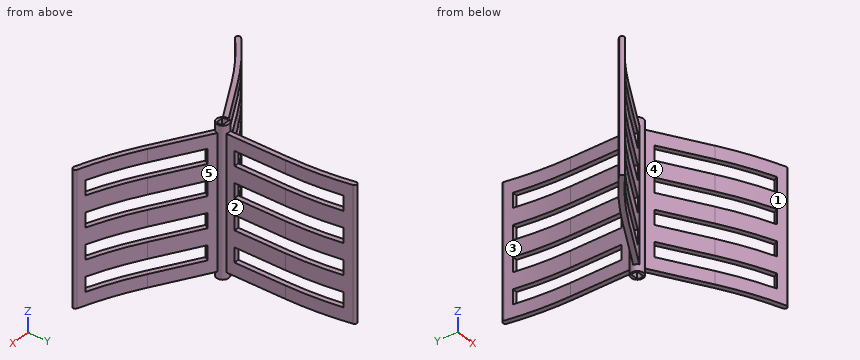
```python
from build123d import *

# Parameters (mm, degrees)
SKETCH_1_R               = 3.75
EXTRUDE_1_DEPTH          = 91
CUT_EXTRUDE_1_DEPTH      = 9
SKETCH_4_R               = 2.5
EXTRUDE_2_DEPTH          = 6
EXTRUDE_START            = -4
EXTRUDE_3_DEPTH          = 82
SKETCH_10_R              = 2.5
EXTRUDE_4_DEPTH          = 2
EXTRUDE_START_2          = 3
EXTRUDE_5_DEPTH          = 3
EXTRUDE_START_3          = 1.5
EXTRUDE_6_DEPTH          = 1.5
CUT_EXTRUDE_4_DEPTH      = 0.5
CUT_EXTRUDE_START        = -8
SKETCH_14_R              = 2.5
CUT_EXTRUDE_5_DEPTH      = 8
CUT_EXTRUDE_9_DEPTH      = 8
CUT_EXTRUDE_10_REACH     = 123.353
SKETCH_16_W              = 9
SKETCH_16_H              = 65
PATTERN_CIRCULAR_1_COUNT = 3
PATTERN_CIRCULAR_2_COUNT = 3


with BuildPart() as part:
    # Sketch 1 → Extrude 1 (new body)
    with BuildSketch(Plane.XY):
        Circle(SKETCH_1_R)
    extrude(amount=EXTRUDE_1_DEPTH)

    # Sketch 2 → Cut-Extrude 1 (cut)
    with BuildSketch(Plane(origin=(0, 0, 0), x_dir=(-1, 0, 0), z_dir=(0, 0, -1))):
        with BuildLine():
            Line((-2, 1.887458609), (2, 1.887458609))
            ThreePointArc((2, 1.887458609), (2.75, 0), (2, -1.887458609))
            Line((2, -1.887458609), (-2, -1.887458609))
            ThreePointArc((-2, -1.887458609), (-2.75, 0), (-2, 1.887458609))
        make_face()
    extrude(amount=-CUT_EXTRUDE_1_DEPTH, mode=Mode.SUBTRACT)

    # Sketch 4 → Extrude 2 (add)
    with BuildSketch(Plane.XY.offset(91)):
        Circle(SKETCH_4_R)
    extrude(amount=EXTRUDE_2_DEPTH)

    # Sketch 7 → Extrude 3 (add)
    with BuildSketch(Plane(origin=(0, 0, 0), x_dir=(-1, 0, 0), z_dir=(0, 0, -1)).offset(EXTRUDE_START)):
        with BuildLine():
            ThreePointArc((-1.5, 3.436931771), (-0.766161164, 3.670898673), (0, 3.75))
            ThreePointArc((0, 3.75), (0.766161164, 3.670898673), (1.5, 3.436931771))
            Line((1.5, 3.436931771), (1.5, 40))
            ThreePointArc((1.5, 40), (2.430132962, 59.193687469), (5.211814999, 78.207499055))
            ThreePointArc((5.211814999, 78.207499055), (5.212182881, 78.20937453), (5.212550781, 78.21125))
            ThreePointArc((5.212550781, 78.21125), (4.02935532, 79.97194546), (2.26865986, 78.78875))
            ThreePointArc((2.26865986, 78.78875), (-0.555622008, 59.485699395), (-1.5, 40))
            Line((-1.5, 40), (-1.5, 3.436931771))
        make_face()
    extrude_3 = extrude(amount=-EXTRUDE_3_DEPTH)

    # Sketch 10 → Extrude 4 (add)
    with BuildSketch(Plane.XY.offset(97)):
        Circle(SKETCH_10_R)
    extrude(amount=EXTRUDE_4_DEPTH)

    # Sketch 11 → Extrude 5 (add)
    with BuildSketch(Plane(origin=(0, 0, 9), x_dir=(-1, 0, 0), z_dir=(0, 0, -1)).offset(EXTRUDE_START_2)):
        with BuildLine():
            Line((-2, -1.887458609), (2, -1.887458609))
            ThreePointArc((2, -1.887458609), (2.75, 0), (2, 1.887458609))
            Line((2, 1.887458609), (-2, 1.887458609))
            ThreePointArc((-2, 1.887458609), (-2.75, 0), (-2, -1.887458609))
        make_face()
    extrude(amount=-EXTRUDE_5_DEPTH)

    # Sketch 12 → Extrude 6 (add)
    with BuildSketch(Plane(origin=(0, 0, 6), x_dir=(-1, 0, 0), z_dir=(0, 0, -1)).offset(EXTRUDE_START_3)):
        with BuildLine():
            Line((-2, -1.887458609), (2, -1.887458609))
            ThreePointArc((2, -1.887458609), (2.75, 0), (2, 1.887458609))
            Line((2, 1.887458609), (-2, 1.887458609))
            ThreePointArc((-2, 1.887458609), (-2.75, 0), (-2, -1.887458609))
        make_face()
    extrude(amount=-EXTRUDE_6_DEPTH)

    # Sketch 13 → Cut-Extrude 4 (cut)
    with BuildSketch(Plane(origin=(0, 0, 4.5), x_dir=(-1, 0, 0), z_dir=(0, 0, -1))):
        with BuildLine():
            Line((-2, -1.887458609), (2, -1.887458609))
            ThreePointArc((2, -1.887458609), (2.75, 0), (2, 1.887458609))
            Line((2, 1.887458609), (-2, 1.887458609))
            ThreePointArc((-2, 1.887458609), (-2.75, 0), (-2, -1.887458609))
        make_face()
    extrude(amount=-CUT_EXTRUDE_4_DEPTH, mode=Mode.SUBTRACT)

    # Sketch 14 → Cut-Extrude 5 (cut)
    with BuildSketch(Plane.XY.offset(99).offset(CUT_EXTRUDE_START)):
        Circle(SKETCH_14_R)
    extrude(amount=CUT_EXTRUDE_5_DEPTH, mode=Mode.SUBTRACT)

    # Sketch 15 → Cut-Extrude 9 (cut)
    with BuildSketch(Plane.XY.offset(91).offset(CUT_EXTRUDE_START)):
        with BuildLine():
            Line((-2, -1.887458609), (2, -1.887458609))
            ThreePointArc((2, -1.887458609), (2.75, 0), (2, 1.887458609))
            Line((2, 1.887458609), (-2, 1.887458609))
            ThreePointArc((-2, 1.887458609), (-2.75, 0), (-2, -1.887458609))
        make_face()
    extrude(amount=CUT_EXTRUDE_9_DEPTH, mode=Mode.SUBTRACT)

    # Sketch 16 → Cut-Extrude 10 (cut, up to next)
    with BuildSketch(Plane(origin=(1.5, 0, 0), x_dir=(0, 0, -1), z_dir=(1, 0, 0)), mode=Mode.PRIVATE) as cut_extrude_10_sk1:
        with Locations((-73.5, 40.936931771)):
            Rectangle(SKETCH_16_W, SKETCH_16_H)
    cut_extrude_10_tool1 = extrude(cut_extrude_10_sk1.sketch, amount=-CUT_EXTRUDE_10_REACH, mode=Mode.PRIVATE) & part.part
    # Sketch 16 → Cut-Extrude 10 (cut, up to next)
    with BuildSketch(Plane(origin=(1.5, 0, 0), x_dir=(0, 0, -1), z_dir=(1, 0, 0)), mode=Mode.PRIVATE) as cut_extrude_10_sk2:
        with Locations((-54.5, 40.936931771)):
            Rectangle(SKETCH_16_W, SKETCH_16_H)
    cut_extrude_10_tool2 = extrude(cut_extrude_10_sk2.sketch, amount=-CUT_EXTRUDE_10_REACH, mode=Mode.PRIVATE) & part.part
    # Sketch 16 → Cut-Extrude 10 (cut, up to next)
    with BuildSketch(Plane(origin=(1.5, 0, 0), x_dir=(0, 0, -1), z_dir=(1, 0, 0)), mode=Mode.PRIVATE) as cut_extrude_10_sk3:
        with Locations((-35.5, 40.936931771)):
            Rectangle(SKETCH_16_W, SKETCH_16_H)
    cut_extrude_10_tool3 = extrude(cut_extrude_10_sk3.sketch, amount=-CUT_EXTRUDE_10_REACH, mode=Mode.PRIVATE) & part.part
    # Sketch 16 → Cut-Extrude 10 (cut, up to next)
    with BuildSketch(Plane(origin=(1.5, 0, 0), x_dir=(0, 0, -1), z_dir=(1, 0, 0)), mode=Mode.PRIVATE) as cut_extrude_10_sk4:
        with Locations((-16.5, 40.936931771)):
            Rectangle(SKETCH_16_W, SKETCH_16_H)
    cut_extrude_10_tool4 = extrude(cut_extrude_10_sk4.sketch, amount=-CUT_EXTRUDE_10_REACH, mode=Mode.PRIVATE) & part.part
    cut_extrude_10_1 = cut_extrude_10_tool1.solids().sort_by_distance((1.5, 40.936932, 73.5))[0]
    add(cut_extrude_10_1, mode=Mode.SUBTRACT)
    cut_extrude_10_2 = cut_extrude_10_tool2.solids().sort_by_distance((1.5, 40.936932, 54.5))[0]
    add(cut_extrude_10_2, mode=Mode.SUBTRACT)
    cut_extrude_10_3 = cut_extrude_10_tool3.solids().sort_by_distance((1.5, 40.936932, 35.5))[0]
    add(cut_extrude_10_3, mode=Mode.SUBTRACT)
    cut_extrude_10_4 = cut_extrude_10_tool4.solids().sort_by_distance((1.5, 40.936932, 16.5))[0]
    add(cut_extrude_10_4, mode=Mode.SUBTRACT)
    cut_extrude_10 = cut_extrude_10_1 + cut_extrude_10_2 + cut_extrude_10_3 + cut_extrude_10_4  # Cut-Extrude 10 as one shape, for the pattern or mirror that repeats it

    # Pattern Circular 1: Extrude 3 ×3 about axis
    pattern_circular_1_axis = Axis((0, 0, 0), (0, 0, 1))
    for i in range(1, PATTERN_CIRCULAR_1_COUNT):
        add(extrude_3.rotate(pattern_circular_1_axis, i * 360 / PATTERN_CIRCULAR_1_COUNT))

    # Pattern Circular 2: Cut-Extrude 10 ×3 about axis
    pattern_circular_2_axis = Axis((0, 0, 0), (0, 0, 1))
    for i in range(1, PATTERN_CIRCULAR_2_COUNT):
        add(cut_extrude_10.rotate(pattern_circular_2_axis, i * 360 / PATTERN_CIRCULAR_2_COUNT), mode=Mode.SUBTRACT)


solid = part.part
```
CAD build for the part. Positions are in the model's coordinates, mm. Face numbers are marked on the shaded views. A direction names the side the tool comes from. Coordinates: 2 decimals unless noted, no trailing zeros. Order: outer loops, then holes, each group sorted by start corner. A loop starts at its lowest first (then second) coordinate and runs counter-clockwise, first axis right, second up.
(1) Mould opens along X. For the marked faces 3, 4 and 5 say: released by +X, released by -X, zero draft, split by the parting line, or undercut.
Solution:
face 3: released by -X
face 4: undercut
face 5: released by +X
(2) Saw through at A-A, the plane z = 38. Count the separate pieces of the cut face and the enclosed holes in it, and give its area (3 significant figures).
Solution:
separate pieces: 4
enclosed holes: 0
area: 144 mm2
(3) Drill centre lines: L1, parallel to Z at x = -41.5, y = -25.5; L2, parallel to X at y = -21, z = 43.5; L3, parallel to X at y = -27, z = 44. Where is each one in solid material? Low to high.
Solution:
L1: z = 4 to 12, 21 to 31, 40 to 50, 59 to 69, 78 to 86
L2: x = -39.27 to -33.37, 33.37 to 39.48
L3: x = -48.56 to -43.17, 44.48 to 51.4
(4) Saw through at B-B, the plane y = 29.5. Write the cut outline in (x, z).
Solution:
outline: (-1.5, 4) - (1.5, 4) - (1.5, 12) - (-1.5, 12) - close; (-1.5, 21) - (1.5, 21) - (1.5, 31) - (-1.5, 31) - close; (-1.5, 40) - (1.5, 40) - (1.5, 50) - (-1.5, 50) - close; (-1.5, 59) - (1.5, 59) - (1.5, 69) - (-1.5, 69) - close; (-1.5, 78) - (1.5, 78) - (1.5, 86) - (-1.5, 86) - close
(5) Saw through at C-C, the plane x = -11. Write the cut outline in (y, z), and give its area (3 significant figures).
Solution:
outline: (-8.08, 4) - (-4.62, 4) - (-4.62, 12) - (-8.08, 12) - close; (-8.08, 21) - (-4.62, 21) - (-4.62, 31) - (-8.08, 31) - close; (-8.08, 40) - (-4.62, 40) - (-4.62, 50) - (-8.08, 50) - close; (-8.08, 59) - (-4.62, 59) - (-4.62, 69) - (-8.08, 69) - close; (-8.08, 78) - (-4.62, 78) - (-4.62, 86) - (-8.08, 86) - close
area: 159 mm2
(6) Which spindle directions (+Z, -Z, +X, -X, +Y, -Y) get a long thin tool onto all of the face, cutting with end or side? Do the marked faces 1 and 2. Say none if no direction does.
Solution:
face 1: +Z, -Z, -Y
face 2: +Z, -Z, +X, +Y
(7) Pin check, flat tips, straight feed: pin 1 Ø2.5 at (x, z) = (0, 34) entering from +Y; pin 2 Ø5 at (x, z) = (-20.5, 63.5) entering from +Y; pin 3 Ø10 at (y, z) = (52, 52) entering from -X. Stop position of each tip, or through.
Solution:
pin 1: stops at y = 8.44
pin 2: stops at y = -8.66
pin 3: stops at x = -2.19
